Autodesk Fusion 360 part; units mm, degrees
sketch "Boceto1" plane through (0, 0, 0) normal (1, 0, 0) x (0, 1, 0)
  arc A0 (50, 0) -> (-50, 0) centre (0, 0) ccw
  line L0 (50, 0) -> (65, 0)
  line L1 (-50, 0) -> (-65, 0)
  arc A1 (65, 0) -> (-65, 0) centre (0, 0) ccw
  dimension "d3" = 100
  dimension "d27" = 15
  dimension "d28" = 15
extrude "Extruir1" add sketch "Boceto1" along normal mid plane 200
sketch "Boceto4" plane through (106.6931, 0, 65) normal (0, 0, 1) x (1, 0, 0)
ref_plane "PlanoDeObra4" through (0, 0, 65) normal (0, 0, 1) x (0, -1, 0)
sketch "Boceto5" plane through (0, 0, 65) normal (0, 0, 1) x (1, 0, 0)
  line L0 (85, 15) -> (-85, 15)
  line L1 (-85, 15) -> (-85, -15)
  line L2 (-85, -15) -> (85, -15)
  line L3 (85, -15) -> (85, 15)
  line L4 (85, 15) -> (-85, -15) construction
  line L5 (-85, 15) -> (85, -15) construction
  dimension "d31" = 170
  dimension "d32" = 30
extrude "Extruir3" cut sketch "Boceto5" against normal blind 10
sketch "Boceto6" plane through (0, 0, 55) normal (0, 0, 1) x (-1, 0, 0)
  line L0 (-85, 15) -> (-85, -15)
  line L1 (-85, -15) -> (85, -15)
  line L2 (85, -15) -> (85, 15)
  line L3 (85, 15) -> (-85, 15)
  circle A0 centre (70, 0) radius 10
  circle A1 centre (40, 0) radius 5
  dimension "d35" = 20
  dimension "d36" = 10
  dimension "d37" = 15
  dimension "d38" = 15
  dimension "d39" = 30
hole "Agujero3" at (-40, 0, 55) direction (0, 0, -1) diameter 8.526 depth 2 tip angle 118
hole "Agujero4" at (-70, 0, 55) direction (0, 0, -1) diameter 20 end through all
ref_plane "PlanoDeObra5" through (0, 0, 60.9016) normal (1, 0, 0) x (0, -1, 0)
mirror "Simetría3" about plane through (0, 0, 60.9016) normal (1, 0, 0) of "Agujero3", "Agujero4"
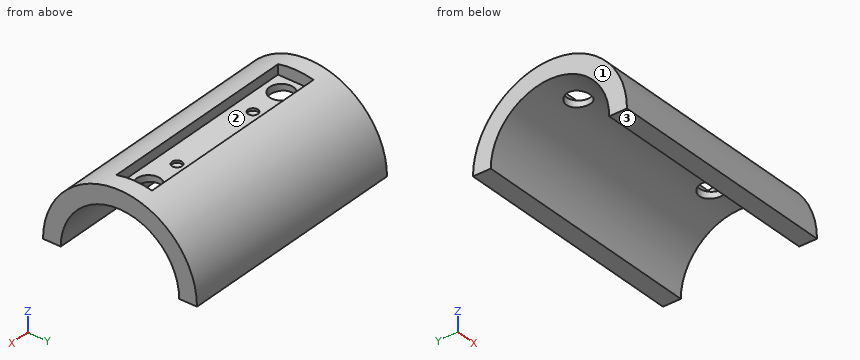
Model file for the job. Use its own axes, mm. Face numbers are marked on the shaded views. Give positions to 0.01 mm unless a question says otherwise; leave off trailing zeros. Order: outer loops, then holes, each group sorted by start corner. A loop starts at its lowest first (then second) coordinate and runs counter-clockwise, first axis right, second up. Notation, with made-up numbers: (-15, 71.25) - (40, 71.25) arc R23 ccw to (40, 103.25) - close; hole circle Ø1 at (-31, 10). An arc over 180 degrees is marked (long way). Write item = value, one per line. Start each with the question number.
1. Cut at D-D, the plane x = 76. List the corners of the cut face in (y, z).
2. Cut at B-B, the plane z = 24.5. List the corners of the cut face in (x, y), and give its area (3 significant figures).
3. Cut at A-A, the plane x = -70. List the corners of the cut face in (y, z).
4. Cut at C-C, the plane y = 6.5. List the corners of the cut face in (x, z).
5. Two-plate mould, pull along X, no slides. Class the marked faces 1, 2 and 3: pulls with the +X half, pulls with the -X half, needs draft (parallel to the pull), parting line crosses it, or undercut.
6. Drop flat-ended pins along their axis: P1, Ø11, axis at x = 40, y = 0, coming from the -Z side; P2, Ø10, axis at x = 30.5, y = -6, coming from the -Z side (3 decimals); P3, Ø1.5, axis at x = 22, z = 37.5, coming from the +Y side. Give the stop position or say it passes through.
7. Probe line 1 along X through (y, z) = (0, 53.25); line 2 along X through (y, z) = (8, 50); line 3 along Y through (x, z) = (70, 53). List the from-to ranges inside material, lowest first.
Taken from the geometry:
q1.outline = (-65, 0) - (-50, 0) arc R50 cw to (-8, 49.36) - (-8, 55) - (-15, 55) - (-15, 63.25) arc R65 ccw to start; (8, 49.36) arc R50 cw to (50, 0) - (65, 0) arc R65 ccw to (15, 63.25) - (15, 55) - (8, 55) - close
q2.outline = (-100, -60.21) - (100, -60.21) - (100, -43.59) - (-100, -43.59) - close; (-100, 43.59) - (100, 43.59) - (100, 60.21) - (-100, 60.21) - close
q2.area = 6,650 mm²
q3.outline = (-65, 0) - (-50, 0) arc R50 cw to (-10, 48.99) - (-10, 55) - (-15, 55) - (-15, 63.25) arc R65 ccw to start; (10, 48.99) arc R50 cw to (50, 0) - (65, 0) arc R65 ccw to (15, 63.25) - (15, 55) - (10, 55) - close
q4.outline = (-100, 49.58) - (-77.6, 49.58) - (-77.6, 55) - (-85, 55) - (-85, 64.67) - (-100, 64.67) - close; (-62.4, 49.58) - (62.4, 49.58) - (62.4, 55) - (-62.4, 55) - close; (77.6, 49.58) - (100, 49.58) - (100, 64.67) - (85, 64.67) - (85, 55) - (77.6, 55) - close
q5.face_1 = pulls with the -X half
q5.face_2 = undercut
q5.face_3 = needs draft
q6.P1 = 49.7
q6.P2 = 48.775
q6.P3 = 53.61
q7.line_1 = -100 to -80, -60 to -44.26, -35.74 to 35.74, 44.26 to 60, 80 to 100
q7.line_2 = -100 to -76, -64 to 64, 76 to 100
q7.line_3 = -37.63 to -10, 10 to 37.63
